Can you work these out from the model? Positions are in its coordinate system, mm. A direction names the side the tool comes from. Coordinates: 2 decimals unless noted, no trailing zeros. Order: outer loops, then holes, each group sorted by start corner. A loop starts at its lowest first (then second) coordinate and runs counter-clockwise, first axis right, second up. Notation, with made-up numbers: (7, 87.5) -> (46, 87.5) arc R19 cw to (46, 102.5) -> close; hole circle Ø2 at (-1.75, 54). An arc over 180 degrees is marked (long way). Write item = value, one per line.
```python
from build123d import *

# Parameters (mm, degrees)
SKETCH1_W               = 900
SKETCH1_H               = 20
SKETCH1_W_2             = 20
SKETCH1_H_2             = 350
SKETCH1_H_3             = 700
BOSS_EXTRUDE1_DEPTH     = 165
CUT_EXTRUDE1_DEPTH      = 2095.283887156
CUT_EXTRUDE1_DEPTH_BACK = 2095.283887156
SKETCH2_W               = 205
SKETCH2_H               = 65
SKETCH2_W_2             = 185
SKETCH2_W_3             = 1800
SKETCH2_H_2             = 20
CUT_EXTRUDE2_DEPTH      = 2095.283887156
CUT_EXTRUDE2_DEPTH_BACK = 2095.283887156
SKETCH3_W               = 200
SKETCH3_H               = 65
SKETCH3_W_2             = 210
SKETCH5_W               = 20
SKETCH5_H               = 780
BOSS_EXTRUDE3_DEPTH     = 40
SCALE2_SCALE            = 0.1


with BuildPart() as part:
    # Sketch1 → Boss-Extrude1 (new body)
    with BuildSketch(Plane(origin=(0, 0, 0), x_dir=(1, 0, 0), z_dir=(0, 1, 0))):
        Polygon((5, 815), (0, 815), (0, 765), (5, 765), (5, 790), align=None)
        with BuildLine():
            Line((5, 790), (5, 765))
            Line((5, 765), (12.32233047, 772.32233047))
            ThreePointArc((12.32233047, 772.32233047), (6.903011687, 780.432914191), (5, 790))
        make_face()
        with BuildLine():
            Line((12.32233047, 772.32233047), (5, 765))
            Line((5, 765), (30, 765))
            ThreePointArc((30, 765), (20.432914191, 766.903011687), (12.32233047, 772.32233047))
        make_face()
        Polygon((5, 765), (0, 765), (0, 760), align=None)
        Polygon((5, 765), (0, 760), (20, 760), (60, 760), (60, 765), (55, 765), (30, 765), align=None)
        with BuildLine():
            Line((55, 765), (55, 790))
            ThreePointArc((55, 790), (47.67766953, 772.32233047), (30, 765))
            Line((30, 765), (55, 765))
        make_face()
        Polygon((60, 800), (60, 820), (55, 815), (55, 790), (55, 765), (60, 765), align=None)
        with BuildLine():
            Line((30, 815), (5, 815))
            Line((5, 815), (5, 790))
            ThreePointArc((5, 790), (12.32233047, 807.67766953), (30, 815))
        make_face()
        Polygon((55, 820), (0, 820), (0, 815), (5, 815), (30, 815), (55, 815), align=None)
        with BuildLine():
            Line((47.67766953, 807.67766953), (55, 815))
            Line((55, 815), (30, 815))
            ThreePointArc((30, 815), (39.567085809, 813.096988313), (47.67766953, 807.67766953))
        make_face()
        with BuildLine():
            Line((55, 790), (55, 815))
            Line((55, 815), (47.67766953, 807.67766953))
            ThreePointArc((47.67766953, 807.67766953), (53.096988313, 799.567085809), (55, 790))
        make_face()
        Polygon((60, 820), (55, 820), (55, 815), align=None)
        with Locations((510, 810)):
            Rectangle(SKETCH1_W, SKETCH1_H)
        with Locations((10, 585)):
            Rectangle(SKETCH1_W_2, SKETCH1_H_2)
        with Locations((10, 235)):
            Rectangle(SKETCH1_W_2, SKETCH1_H_2)
        Polygon((5, 55), (0, 60), (0, 55), align=None)
        Polygon((5, 55), (0, 55), (0, 5), (5, 5), (5, 30), align=None)
        Polygon((20, 60), (0, 60), (5, 55), (30, 55), (55, 55), (60, 55), (60, 60), align=None)
        with BuildLine():
            Line((30, 55), (5, 55))
            Line((5, 55), (12.32233047, 47.67766953))
            ThreePointArc((12.32233047, 47.67766953), (20.432914191, 53.096988313), (30, 55))
        make_face()
        with BuildLine():
            Line((12.32233047, 47.67766953), (5, 55))
            Line((5, 55), (5, 30))
            ThreePointArc((5, 30), (6.903011687, 39.567085809), (12.32233047, 47.67766953))
        make_face()
        with BuildLine():
            Line((55, 55), (30, 55))
            ThreePointArc((30, 55), (47.67766953, 47.67766953), (55, 30))
            Line((55, 30), (55, 55))
        make_face()
        Polygon((60, 0), (60, 20), (60, 55), (55, 55), (55, 30), (55, 5), align=None)
        with BuildLine():
            Line((55, 5), (47.67766953, 12.32233047))
            ThreePointArc((47.67766953, 12.32233047), (39.567085809, 6.903011687), (30, 5))
            Line((30, 5), (55, 5))
        make_face()
        with BuildLine():
            ThreePointArc((55, 30), (53.096988313, 20.432914191), (47.67766953, 12.32233047))
            Line((47.67766953, 12.32233047), (55, 5))
            Line((55, 5), (55, 30))
        make_face()
        Polygon((5, 5), (0, 5), (0, 0), (55, 0), (55, 5), (30, 5), align=None)
        Polygon((55, 0), (60, 0), (55, 5), align=None)
        with BuildLine():
            ThreePointArc((30, 5), (12.32233047, 12.32233047), (5, 30))
            Line((5, 30), (5, 5))
            Line((5, 5), (30, 5))
        make_face()
        with Locations((510, 10)):
            Rectangle(SKETCH1_W, SKETCH1_H)
        with Locations((1410, 10)):
            Rectangle(SKETCH1_W, SKETCH1_H)
        Polygon((1860, 55), (1860, 20), (1860, 0), (1865, 5), (1865, 30), (1865, 55), align=None)
        with BuildLine():
            Line((1865, 30), (1865, 5))
            Line((1865, 5), (1872.32233047, 12.32233047))
            ThreePointArc((1872.32233047, 12.32233047), (1866.903011687, 20.432914191), (1865, 30))
        make_face()
        with BuildLine():
            Line((1872.32233047, 12.32233047), (1865, 5))
            Line((1865, 5), (1890, 5))
            ThreePointArc((1890, 5), (1880.432914191, 6.903011687), (1872.32233047, 12.32233047))
        make_face()
        Polygon((1865, 5), (1860, 0), (1865, 0), align=None)
        Polygon((1865, 5), (1865, 0), (1920, 0), (1920, 5), (1915, 5), (1890, 5), align=None)
        with BuildLine():
            ThreePointArc((1915, 30), (1907.67766953, 12.32233047), (1890, 5))
            Line((1890, 5), (1915, 5))
            Line((1915, 5), (1915, 30))
        make_face()
        Polygon((1920, 5), (1920, 55), (1915, 55), (1915, 30), (1915, 5), align=None)
        Polygon((1860, 60), (1860, 55), (1865, 55), (1890, 55), (1915, 55), (1920, 60), (1900, 60), align=None)
        with BuildLine():
            Line((1890, 55), (1865, 55))
            Line((1865, 55), (1865, 30))
            ThreePointArc((1865, 30), (1872.32233047, 47.67766953), (1890, 55))
        make_face()
        with BuildLine():
            Line((1915, 55), (1890, 55))
            ThreePointArc((1890, 55), (1899.567085809, 53.096988313), (1907.67766953, 47.67766953))
            Line((1907.67766953, 47.67766953), (1915, 55))
        make_face()
        Polygon((1920, 55), (1920, 60), (1915, 55), align=None)
        with BuildLine():
            Line((1915, 30), (1915, 55))
            Line((1915, 55), (1907.67766953, 47.67766953))
            ThreePointArc((1907.67766953, 47.67766953), (1913.096988313, 39.567085809), (1915, 30))
        make_face()
        with Locations((1910, 410)):
            Rectangle(SKETCH1_W_2, SKETCH1_H_3)
        Polygon((1865, 765), (1860, 765), (1860, 760), (1900, 760), (1920, 760), (1915, 765), (1890, 765), align=None)
        Polygon((1920, 760), (1920, 765), (1915, 765), align=None)
        with BuildLine():
            ThreePointArc((1915, 790), (1913.096988313, 780.432914191), (1907.67766953, 772.32233047))
            Line((1907.67766953, 772.32233047), (1915, 765))
            Line((1915, 765), (1915, 790))
        make_face()
        with BuildLine():
            Line((1915, 765), (1907.67766953, 772.32233047))
            ThreePointArc((1907.67766953, 772.32233047), (1899.567085809, 766.903011687), (1890, 765))
            Line((1890, 765), (1915, 765))
        make_face()
        Polygon((1920, 765), (1920, 815), (1915, 815), (1915, 790), (1915, 765), align=None)
        Polygon((1920, 820), (1865, 820), (1865, 815), (1890, 815), (1915, 815), (1920, 815), align=None)
        with BuildLine():
            Line((1915, 815), (1890, 815))
            ThreePointArc((1890, 815), (1907.67766953, 807.67766953), (1915, 790))
            Line((1915, 790), (1915, 815))
        make_face()
        Polygon((1865, 820), (1860, 820), (1865, 815), align=None)
        Polygon((1865, 815), (1860, 820), (1860, 800), (1860, 765), (1865, 765), (1865, 790), align=None)
        with BuildLine():
            Line((1872.32233047, 807.67766953), (1865, 815))
            Line((1865, 815), (1865, 790))
            ThreePointArc((1865, 790), (1866.903011687, 799.567085809), (1872.32233047, 807.67766953))
        make_face()
        with BuildLine():
            Line((1890, 815), (1865, 815))
            Line((1865, 815), (1872.32233047, 807.67766953))
            ThreePointArc((1872.32233047, 807.67766953), (1880.432914191, 813.096988313), (1890, 815))
        make_face()
        with BuildLine():
            ThreePointArc((1890, 765), (1872.32233047, 772.32233047), (1865, 790))
            Line((1865, 790), (1865, 765))
            Line((1865, 765), (1890, 765))
        make_face()
        with Locations((1410, 810)):
            Rectangle(SKETCH1_W, SKETCH1_H)
    extrude(amount=BOSS_EXTRUDE1_DEPTH)

    # Sketch2 → Cut-Extrude1 (cut, two sides: drawn at the far end of the back side and taken through both)
    with BuildSketch(Plane.XY.offset(-CUT_EXTRUDE1_DEPTH_BACK)):
        with Locations((162.5, 72.5)):
            Rectangle(SKETCH2_W, SKETCH2_H)
        with Locations((397.5, 72.5)):
            Rectangle(SKETCH2_W_2, SKETCH2_H)
        with Locations((622.5, 72.5)):
            Rectangle(SKETCH2_W_2, SKETCH2_H)
        with Locations((847.5, 72.5)):
            Rectangle(SKETCH2_W_2, SKETCH2_H)
        with Locations((1072.5, 72.5)):
            Rectangle(SKETCH2_W_2, SKETCH2_H)
        with Locations((1297.5, 72.5)):
            Rectangle(SKETCH2_W_2, SKETCH2_H)
        with Locations((1522.5, 72.5)):
            Rectangle(SKETCH2_W_2, SKETCH2_H)
        with Locations((1757.5, 72.5)):
            Rectangle(SKETCH2_W, SKETCH2_H)
        with Locations((960, 155)):
            Rectangle(SKETCH2_W_3, SKETCH2_H_2)
    extrude(amount=CUT_EXTRUDE1_DEPTH + CUT_EXTRUDE1_DEPTH_BACK, mode=Mode.SUBTRACT)

    # Sketch3 → Cut-Extrude2 (cut, two sides: drawn at the far end of the back side and taken through both)
    with BuildSketch(Plane(origin=(1920, 0, 0), x_dir=(0, 0, -1), z_dir=(1, 0, 0)).offset(-CUT_EXTRUDE2_DEPTH_BACK)):
        Polygon((410, 145), (410, 165), (60, 165), (60, 145), (270, 145), (310, 145), align=None)
        Polygon((760, 145), (760, 165), (410, 165), (410, 145), (510, 145), (550, 145), align=None)
        with Locations((410, 72.5)):
            Rectangle(SKETCH3_W, SKETCH3_H)
        with Locations((655, 72.5)):
            Rectangle(SKETCH3_W_2, SKETCH3_H)
        with Locations((165, 72.5)):
            Rectangle(SKETCH3_W_2, SKETCH3_H)
    extrude(amount=CUT_EXTRUDE2_DEPTH + CUT_EXTRUDE2_DEPTH_BACK, mode=Mode.SUBTRACT)

    # Sketch5 → Boss-Extrude3 (add)
    with BuildSketch(Plane.XZ):
        with Locations((650, -410)):
            Rectangle(SKETCH5_W, SKETCH5_H)
        with Locations((1270, -410)):
            Rectangle(SKETCH5_W, SKETCH5_H)
    extrude(amount=-BOSS_EXTRUDE3_DEPTH)


with BuildPart() as part_1:
    # Scale2: scaled about (960, 67.642168167, -410)
    add(part.part.scale(SCALE2_SCALE).moved(Location((864, 60.87795135, -369))))


solid = part_1.part
```
Item 1: I'm going to push flat-ended pins straight in: P1, Ø2, axis at x = 1018, z = -450, coming from the +Y side; P2, Ø3, axis at x = 930, z = -416, coming from the +Y side. Where does each tip first touch, or does it pass through?
A:
P1 = 75.38
P2 = 64.88
Item 2: If we mould it in two halves opening along Z, with no side actions, what happens to faces 1 (the flat face through (959, 67, -369)), 2 (the flat face through (868, 69, -375)), 3 (the flat face through (867, 77.378, -450.7))? For each: pulls with the +Z half, pulls with the -Z half, needs draft (parallel to the pull), parting line crosses it, or undercut.
A:
face_1 = pulls with the +Z half
face_2 = undercut
face_3 = needs draft
Item 3: I want a section at A-A, the plane z = -409.5. Please give me the cut outline in (x, y).
A:
outline = (864, 60.88) -> (866, 60.88) -> (866, 64.88) -> (864, 64.88) -> close; (864, 71.38) -> (866, 71.38) -> (866, 75.38) -> (864, 75.38) -> close; (928, 60.88) -> (930, 60.88) -> (930, 64.88) -> (928, 64.88) -> close; (990, 60.88) -> (992, 60.88) -> (992, 64.88) -> (990, 64.88) -> close; (1054, 60.88) -> (1056, 60.88) -> (1056, 64.88) -> (1054, 64.88) -> close; (1054, 71.38) -> (1056, 71.38) -> (1056, 75.38) -> (1054, 75.38) -> close
Item 4: If I drill on probe 1 along X at (y, z) = (63.75, -425.5); probe 2 along Z at (x, y) = (980.5, 63.25); probe 3 along X at (y, z) = (73.75, -432), over which ranges is the centre line in solid material (lowest first)?
A:
probe_1 = 864 to 866, 928 to 930, 990 to 992, 1054 to 1056
probe_2 = -451 to -449, -371 to -369
probe_3 = 864 to 866, 1054 to 1056
Item 5: I want a section at C-C, the plane y = 67.5. Give the number of separate pieces and of enclosed holes in the cut face, plus the area to 3 significant figures.
A:
separate_pieces = 22
enclosed_holes = 4
area = 209 mm2
Item 6: I want a section at B-B, the plane x = 998.5. Please give me the cut outline in (y, z).
A:
outline = (60.88, -451) -> (64.88, -451) -> (64.88, -449) -> (60.88, -449) -> close; (60.88, -371) -> (64.88, -371) -> (64.88, -369) -> (60.88, -369) -> close; (71.38, -451) -> (75.38, -451) -> (75.38, -449) -> (71.38, -449) -> close; (71.38, -371) -> (75.38, -371) -> (75.38, -369) -> (71.38, -369) -> close
Item 7: For faces 4 (the flat face through (928, 63, -411)), 5 (the flat face through (1050, 69, -373)), 6 (the flat face through (929.6, 64.878, -410.2)), which set-ups out of +Z, -Z, +X, -X, +Y, -Y let a thin tool reach every point of the face, with its end or its side?
A:
face_4 = +Y, -Y
face_5 = none
face_6 = +Z, -Z
